```python
from build123d import *

# Parameters (mm, degrees)
SKETCH_1_R          = 10
SKETCH_1_R_2        = 3.25
EXTRUDE_1_DEPTH     = 5
SKETCH_2_W          = 10
SKETCH_2_H          = 10
EXTRUDE_4_DEPTH     = 30
CUT_EXTRUDE_START   = -30
SKETCH_6_R          = 3.25
CUT_EXTRUDE_1_DEPTH = 30
SKETCH_7_R          = 1.5
CUT_EXTRUDE_3_DEPTH = 5


with BuildPart() as part:
    # Эскиз1 → Бобышка-Вытянуть1 (new body)
    with BuildSketch(Plane.XY):
        Circle(SKETCH_1_R)
        Circle(SKETCH_1_R_2, mode=Mode.SUBTRACT)
    extrude(amount=EXTRUDE_1_DEPTH)

    # Эскиз2 → Бобышка-Вытянуть4 (add)
    with BuildSketch(Plane.XY.offset(5)):
        Rectangle(SKETCH_2_W, SKETCH_2_H)
    extrude(amount=EXTRUDE_4_DEPTH)

    # Эскиз6 → Вырез-Вытянуть1 (cut)
    with BuildSketch(Plane.XY.offset(35).offset(CUT_EXTRUDE_START)):
        Circle(SKETCH_6_R)
    extrude(amount=CUT_EXTRUDE_1_DEPTH, mode=Mode.SUBTRACT)

    # Эскиз7 → Вырез-Вытянуть3 (cut)
    with BuildSketch(Plane(origin=(0, 5, 0), x_dir=(1, 0, 0), z_dir=(0, 1, 0))):
        with Locations(Location((0, -30, 0), (0, 0, 270))):
            Circle(SKETCH_7_R)
    extrude(amount=-CUT_EXTRUDE_3_DEPTH, mode=Mode.SUBTRACT)


solid = part.part
```
Geometry: final body of the model. Coordinates: model frame, mm. A direction names the side the tool comes from. Give positions to 0.01 mm unless a question says otherwise; leave off trailing zeros. Loops run counter-clockwise (first coordinate to the right, second up) from the corner with the lowest first, then second, coordinate; pieces in that order, holes last. Notation, with made-up numbers: (83.5, 87) -> (114.5, 87) arc R19 ccw to (114.5, 124) -> close; hole circle Ø9 at (60, 67). An arc over 180 degrees is marked (long way). Return JSON: item names as keys, results as strings.
Item 1: Section D-D, the plane z = 21. Output: boundary loops of the cut face in (x, y), plus the area to 3 significant figures.
Filled in:
{"outline": "(-5, -5) -> (5, -5) -> (5, 5) -> (-5, 5) -> close; hole circle Ø6.5 at (0, 0)", "area": "66.8 mm^2"}
Item 2: Section A-A, the plane x = 0. Output: boundary loops of the cut face in (y, z), plus the area to 3 significant figures.
Filled in:
{"outline": "(-10, 0) -> (-3.25, 0) -> (-3.25, 35) -> (-5, 35) -> (-5, 5) -> (-10, 5) -> close; (3.25, 0) -> (10, 0) -> (10, 5) -> (5, 5) -> (5, 28.5) -> (3.25, 28.5) -> close; (3.25, 31.5) -> (5, 31.5) -> (5, 35) -> (3.25, 35) -> close", "area": "167 mm^2"}
Item 3: Pin query (flat end, axial travel): P1, Ø12, axis at x = -7.5, z = 24.5, coming from the -Y side; P2, Ø5, axis at y = -1.5, z = 19, coming from the +X side; P3, Ø3, axis at x = -0.5, z = 19, coming from the +Y side. Return the tip coordinate at first contact, or that it passes through.
Filled in:
{"P1": "y = -5", "P2": "x = 5", "P3": "y = 5"}
Item 4: Mould query, pull axis X, two halves, no side actions, for faces 5 (the flat face through (-5, 0, 20)), 6 (the cylindrical face through (-2.17, -9.76, 2.46)), 7 (the flat face through (-0.1, 3.4, 35)), 8 (the cylindrical face through (0.45, 3.96, 31.43)). Classes: released by +X, released by -X, zero draft, split by the parting line, or undercut.
Filled in:
{"face 5": "released by -X", "face 6": "split by the parting line", "face 7": "zero draft", "face 8": "undercut"}
Item 5: Access query for faces 1 (the flat face through (0, -5, 20)), 2 (the flat face through (5, 0, 20)), 3 (the cylindrical face through (-0.705, -3.173, 17.255)), 4 (the flat face through (0, 5, 20)). Directions: +Z, -Z, +X, -X, +Y, -Y. A direction counts if a zero-diameter tool reaches every point of the face in a straight line with its end or side. Return the directions, or none.
Filled in:
{"face 1": "+Z, +X, -X, -Y", "face 2": "+Z, +X, +Y, -Y", "face 3": "+Z, -Z", "face 4": "+Z, +X, -X, +Y"}
Item 6: Section B-B, the plane y = 0. Output: boundary loops of the cut face in (x, z), plus the area to 4 significant figures.
Filled in:
{"outline": "(-10, 0) -> (-3.25, 0) -> (-3.25, 35) -> (-5, 35) -> (-5, 5) -> (-10, 5) -> close; (3.25, 0) -> (10, 0) -> (10, 5) -> (5, 5) -> (5, 35) -> (3.25, 35) -> close", "area": "172.5 mm^2"}
Item 7: Line query: line 1 (Z direction, x = 0, y = 4.65); line 2 (Y direction, x = 0, z = 13); line 3 (X direction, y = 4.05, z = 30). Output: solid intervals per line, ascending.
Filled in:
{"line 1": "0 to 28.5, 31.5 to 35", "line 2": "-5 to -3.25, 3.25 to 5", "line 3": "-5 to -1.5, 1.5 to 5"}
Item 8: Section C-C, the plane x = 2. Output: boundary loops of the cut face in (y, z), plus the area to 3 significant figures.
Filled in:
{"outline": "(-9.8, 0) -> (-2.56, 0) -> (-2.56, 35) -> (-5, 35) -> (-5, 5) -> (-9.8, 5) -> close; (2.56, 0) -> (9.8, 0) -> (9.8, 5) -> (5, 5) -> (5, 35) -> (2.56, 35) -> close", "area": "219 mm^2"}
